Here's the drawing with two shaded views (mm, measured from the low corner). I have some questions. A direction names the side the tool comes from. Round coordinates to 2 decimals unless told otherwise and drop trailing zeros. Order: outer loops, then holes, each group sorted by start corner. A loop starts at its lowest first (then second) coordinate and runs counter-clockwise, first axis right, second up. Notation, with made-up numbers: (65.25, 76) -> (124.25, 76) arc R19 cw to (124.25, 99) -> close; hole circle Ø5 at (22, 59.5). An arc over 180 degrees is marked (long way). Put each result on its own line as item: value. Start each with the question number.
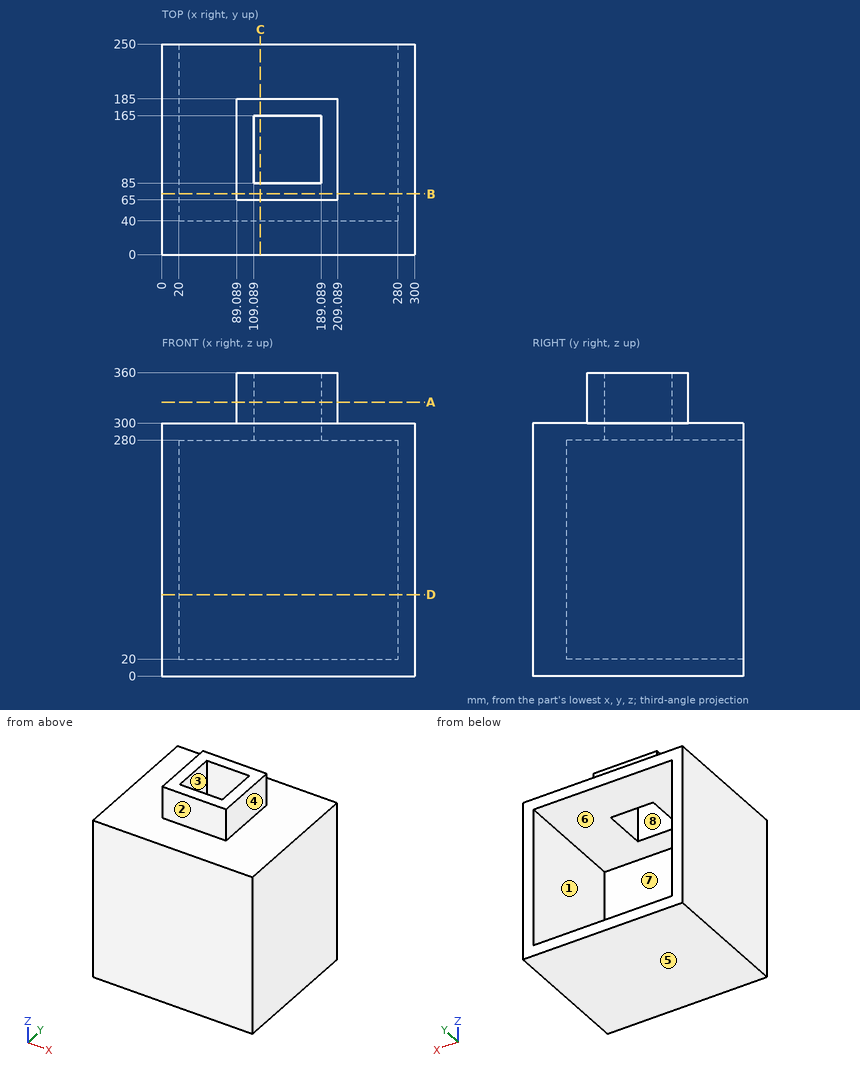
1. If we section it at C-C, the plane x = 117: Please give me the cut outline in (y, z), then the cut area to 3 significant figures.
2. Thinking about a two-plate mould opening in Z: for the marked faces 5, 6, 7 and 8, which applies, +Z half, -Z half, draft (parallel to the pull), parting line (faces both ways), or undercut?
3. For pin 1 Ø3 at (x, z) = (175, 320) entering from +Y; pin 2 Ø24 at (y, z) = (139.5, 319) entering from -X, each with a flat end and sliding along its axis, tell me the tip position at first contact or that it passes through.
4. If we section it at B-B, the plane y = 72: Please give me the cut outline in (x, z).
5. Which directions (+Z, -Z, +X, -X, +Y, -Y) give clear straight access to the entire face, cutting with the end or side of a thin tool? Please do the marked faces 1, 2, 3 and 4.
6. If we section it at D-D, the plane z = 96.5: Please give me the cut outline in (x, y), then the cut area to 3 significant figures.
7. If we section it at A-A, the plane z = 325: Please give me the cut outline in (x, y).
8. I need wall thicknesses on L1, parallel to Z at x = 66.5, y = 118.5; L2, parallel to Y at x = 186, z = 23.5. Which ranges of each line are inside material? Lowest first, please.
Results below:
1. outline: (0, 0) -> (250, 0) -> (250, 20) -> (40, 20) -> (40, 280) -> (85, 280) -> (85, 360) -> (65, 360) -> (65, 300) -> (0, 300) -> close; (165, 280) -> (250, 280) -> (250, 300) -> (185, 300) -> (185, 360) -> (165, 360) -> close
1. area: 21,200 mm2
2. face 5: -Z half
2. face 6: undercut
2. face 7: undercut
2. face 8: draft
3. pin 1: y = 185
3. pin 2: x = 89.09
4. outline: (0, 0) -> (300, 0) -> (300, 300) -> (209.09, 300) -> (209.09, 360) -> (89.09, 360) -> (89.09, 300) -> (0, 300) -> close; hole (20, 20) -> (280, 20) -> (280, 280) -> (20, 280) -> close
5. face 1: +Y
5. face 2: +Z, +X, -X, -Y
5. face 3: +Z
5. face 4: +Z, +X, +Y, -Y
6. outline: (0, 0) -> (300, 0) -> (300, 250) -> (280, 250) -> (280, 40) -> (20, 40) -> (20, 250) -> (0, 250) -> close
6. area: 20,400 mm2
7. outline: (89.09, 65) -> (209.09, 65) -> (209.09, 185) -> (89.09, 185) -> close; hole (109.09, 85) -> (189.09, 85) -> (189.09, 165) -> (109.09, 165) -> close
8. L1: 0 to 20, 280 to 300
8. L2: 0 to 40
